Here's how the part is built. I have some questions about the finished solid (model axes, mm). Face numbers are marked on the shaded views. A direction names the side the tool comes from. Round coordinates to 2 decimals unless told otherwise and drop trailing zeros. Loops run counter-clockwise (first coordinate to the right, second up) from the corner with the lowest first, then second, coordinate; pieces in that order, holes last. Notation, with made-up numbers: M 19,44.5 L 77,44.5 A23 cw 77,74.5 Z; hole C 80,19 d2. An arc over 180 degrees is marked long. Answer as a JSON object with one key per item and string values.
Autodesk Inventor part; units mm, degrees
ref_plane "YZ Plane" through (0, 0, 0) normal (1, 0, 0) x (0, 1, 0)
ref_plane "XZ Plane" through (0, 0, 0) normal (0, 1, 0) x (-1, 0, 0)
ref_plane "XY Plane" through (0, 0, 0) normal (0, 0, 1) x (1, 0, 0)
sketch "Sketch1" plane through (0, 0, 0) normal (0, 1, 0) x (-1, 0, 0)
  line L0 (10.5, 0) -> (-10.5, 0)
  line L1 (0, -42) -> (0, 42)
  line L2 (7.5, -30) -> (-7.5, -30)
  line L3 (-7.5, -30) -> (-7.5, 30)
  line L4 (-7.5, 30) -> (7.5, 30)
  line L5 (7.5, 30) -> (7.5, -30)
  point P0 (0, 0)
  dimension "d0" = 15
  dimension "d1" = 60
extrude "Extrusion1" add sketch "Sketch1" along normal blind 3
sketch "Sketch2" plane through (0, 3, 0) normal (0, 1, 0) x (1, 0, 0)
  line L0 (7.5, 30) -> (-7.5, 30)
  line L1 (-7.5, 30) -> (-7.5, -30)
  line L2 (-7.5, -30) -> (7.5, -30)
  line L3 (7.5, -30) -> (7.5, 30)
  circle A0 centre (0, -22) radius 3.75
  circle A1 centre (0, -8) radius 2.5
  line L4 (0, 42) -> (0, -42)
  line L5 (-7.5, -5.5) -> (7.5, -5.5) construction
  line L6 (-2.4495, -7.5) -> (-3.75, -22)
  line L7 (3.75, -22) -> (2.4495, -7.5)
  line L8 (-10.5, 0) -> (10.5, 0)
  circle A2 centre (0, 22) radius 3.75
  circle A3 centre (0, 8) radius 2.5
  line L9 (-2.4495, 7.5) -> (-3.75, 22)
  line L10 (3.75, 22) -> (2.4495, 7.5)
  point P0 (0, 0)
  dimension "d4" = 7.5
  dimension "d5" = 8
  dimension "d6" = 5
  dimension "d9" = 16.5
  dimension "d10" = 2
  dimension "d11" = 8
  dimension "d12" = 8
  dimension "d13" = 2
extrude "Extrusion2" cut sketch "Sketch2" against normal blind 2 contours A2 L10 L4 | L4 A2 L9 | A2 L10 A3 L4 | L4 A3 L9 A2 | A3 L9 L4 | L4 A3 L10 | L4 A1 L6 | A1 L7 L4 | L4 A0 L7 | A0 L6 L4 | A1 L7 | L6 A1 | L4 A0 L6 A1 | A1 L7 A0 L4
sketch "Sketch3" plane through (0, 1, 0) normal (0, 1, 0) x (1, 0, 0)
  line L0 (7.5, 30) -> (-7.5, 30)
  line L1 (-7.5, 30) -> (-7.5, -30)
  line L2 (-7.5, -30) -> (7.5, -30)
  line L3 (7.5, -30) -> (7.5, 30)
  line L4 (-3.75, -22) -> (-2.4994, -8.0561)
  arc A0 (-3.75, -22) -> (3.75, -22) centre (0, -22) ccw
  line L5 (2.4994, -8.0561) -> (3.75, -22)
  arc A1 (2.4994, -8.0561) -> (-2.4994, -8.0561) centre (0, -8) ccw
  line L6 (3.75, 22) -> (2.4495, 7.5)
  arc A2 (3.75, 22) -> (-3.75, 22) centre (0, 22) ccw
  line L7 (-2.4495, 7.5) -> (-3.75, 22)
  arc A3 (-2.4495, 7.5) -> (2.4495, 7.5) centre (0, 8) ccw
  line L8 (-10.5, 0) -> (10.5, 0)
  point P0 (0, 0)
hole "Hole1" at (0, 1, 22) at (0, 1, -22) direction (0, -1, 0) diameter 7.5 end through all
fillet "Fillet1" radius 6 4 edges at (7.5, 1.5, -30) (-7.5, 1.5, -30) (-7.5, 1.5, 30) (7.5, 1.5, 30)
sketch "Sketch5" plane through (0, 3, 0) normal (0, 1, 0) x (1, 0, 0)
  arc A0 (3.75, 22) -> (-3.75, 22) centre (0, 22) ccw
  line L0 (3.75, 22) -> (2.4495, 7.5)
  arc A1 (-2.4495, 7.5) -> (2.4495, 7.5) centre (0, 8) ccw
  line L1 (-2.4495, 7.5) -> (-3.75, 22)
  line L2 (-3.75, -22) -> (-2.4994, -8.0561)
  arc A2 (2.4994, -8.0561) -> (-2.4994, -8.0561) centre (0, -8) ccw
  line L3 (2.4994, -8.0561) -> (3.75, -22)
  arc A3 (-3.75, -22) -> (3.75, -22) centre (0, -22) ccw
  arc A4 (1.5, -30) -> (7.5, -24) centre (1.5, -24) ccw
  line L4 (7.5, -24) -> (7.5, 24)
  arc A5 (7.5, 24) -> (1.5, 30) centre (1.5, 24) ccw
  line L5 (1.5, 30) -> (-1.5, 30)
  arc A6 (-1.5, 30) -> (-7.5, 24) centre (-1.5, 24) ccw
  line L6 (-7.5, 24) -> (-7.5, -24)
  arc A7 (-7.5, -24) -> (-1.5, -30) centre (-1.5, -24) ccw
  line L7 (-1.5, -30) -> (1.5, -30)
  point P0 (0, 0)
  point P1 (0, 0)
hole "Hole3" at (0, 3, 0) direction (0, -1, 0) diameter 4 end through all
properties part number "femur_v5"
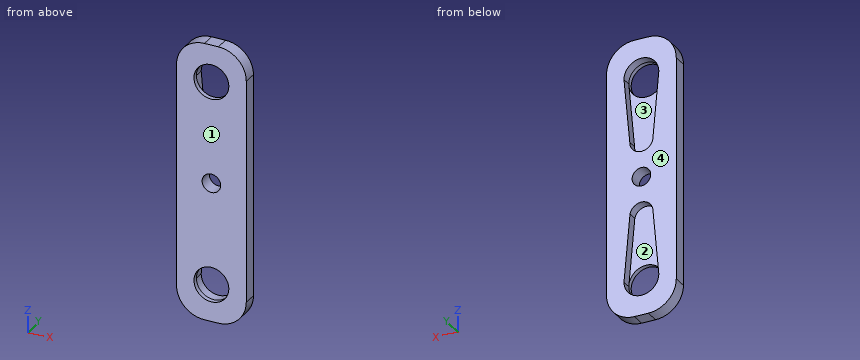
Item 1: On a 3-axis mill with a long thin cutter (end or side, diameter ignored), from which of +Z, -Z, +X, -X, +Y, -Y can I reach the whole of each face in a straight line? I mean the marked faces 1 and 2. Say none if no direction works.
Resolved:
{"face 1": "+Z, -Z, +X, -X, -Y", "face 2": "+Y"}
Item 2: I want a section at B-B, the plane y = 2.2. Please give me the cut outline in (x, z).
Resolved:
{"outline": "M -7.5,-24 A6 ccw -1.5,-30 L 1.5,-30 A6 ccw 7.5,-24 L 7.5,24 A6 ccw 1.5,30 L -1.5,30 A6 ccw -7.5,24 Z; hole M -3.75,-22 A3.75 ccw 3.75,-22 L 2.45,-7.5 A2.5 ccw -2.45,-7.5 Z; hole M -3.75,22 L -2.5,8.06 A2.5 ccw long 2.5,8.06 L 3.75,22 A3.75 ccw Z; hole C 0,0 d4"}
Item 3: I want a section at A-A, the plane z = 0. Please give me the cut outline in (x, y).
Resolved:
{"outline": "M -7.5,0 L -2,0 L -2,3 L -7.5,3 Z; M 2,0 L 7.5,0 L 7.5,3 L 2,3 Z"}
Item 4: If we mould it in two halves opening along X, with no side actions, what happens to the marked faces 3 and 4? For each: pulls with the +X half, pulls with the -X half, needs draft (parallel to the pull), parting line crosses it, or undercut.
Resolved:
{"face 3": "undercut", "face 4": "needs draft"}
Item 5: I'm going to push flat-ended pins straight in: pin 1 Ø1.5 at (x, y) = (4.5, 1) entering from +Z; pin 2 Ø5 at (x, z) = (-0.5, -19) entering from +Y. Where does each tip first touch, or does it pass through?
Resolved:
{"pin 1": "z = 29.56", "pin 2": "y = 1"}
Item 6: I want a section at D-D, the plane x = 5.5. Please give me the cut outline in (y, z), then the cut area to 3 significant figures.
Resolved:
{"outline": "M 0,-28.47 L 3,-28.47 L 3,28.47 L 0,28.47 Z", "area": "171 mm²"}
Item 7: Please list where these lines run through material, in increasing order: probe 1 along Z at (x, y) = (0, 1.3); probe 2 along Z at (x, y) = (0, 0.35); probe 3 along Z at (x, y) = (-2.25, 2.6). Write a range as from..to.
Resolved:
{"probe 1": "-30..-25.75, -5.5..-2, 2..5.5, 25.75..30", "probe 2": "-30..-25.75, -18.25..-2, 2..18.25, 25.75..30", "probe 3": "-29.95..-25, -6.91..6.91, 25..29.95"}
Item 8: I want a section at C-C, the plane x = 0. Please give me the cut outline in (y, z), then the cut area to 3 significant figures.
Resolved:
{"outline": "M 0,-30 L 3,-30 L 3,-25.75 L 0,-25.75 Z; M 0,-18.25 L 1,-18.25 L 1,-5.5 L 3,-5.5 L 3,-2 L 0,-2 Z; M 0,2 L 3,2 L 3,5.5 L 1,5.5 L 1,18.25 L 0,18.25 Z; M 0,25.75 L 3,25.75 L 3,30 L 0,30 Z", "area": "72.0 mm²"}
